```python
from build123d import *

# Parameters (mm, degrees)
F0_W     = 16
F0_H     = 8
F1_DEPTH = 8
F2_W     = 16
F2_H     = 3
F3_DEPTH = 33.2
F4_W     = 19
F4_H     = 3
F5_DEPTH = 12
F6_R     = 2
F7_DEPTH = 3
F8_W     = 16
F8_H     = 3
F9_DEPTH = 6
F10_R    = 1.99999


# Not quite as in the source:
# - a fillet or chamfer is up to 0.001 mm smaller than in the source, because OpenCascade refuses the exact size


with BuildPart() as f1:
    # F0 (on Top) → F1 (new body)
    with BuildSketch(Plane.XY):
        with Locations((-8, 4)):
            Rectangle(F0_W, F0_H)
    extrude(amount=F1_DEPTH)

    # F2 (on Top) → F3 (join)
    with BuildSketch(Plane.XY):
        with Locations((-8, -1.5)):
            Rectangle(F2_W, F2_H)
        Polygon((0, 6), (0, 0), (0, -3), (3, -3), (3, 6), align=None)
    extrude(amount=F3_DEPTH)

    # F4 (on face) → F5 (join)
    with BuildSketch(Plane.XZ.offset(3)):
        with Locations((-6.5, 1.5)):
            Rectangle(F4_W, F4_H)
    extrude(amount=F5_DEPTH)

    # F6 (on face) → F7 (cut, through all)
    with BuildSketch(Plane.XY.offset(3)):
        with Locations((-6.3249543309, -9.8292976618)):
            Circle(F6_R)
    extrude(amount=-F7_DEPTH, mode=Mode.SUBTRACT)

    # F8 (on face) → F9 (join)
    with BuildSketch(Plane(origin=(0, 0, 0), x_dir=(-1, 0, 0), z_dir=(0, 1, 0))):
        with Locations((8, 31.7)):
            Rectangle(F8_W, F8_H)
    extrude(amount=F9_DEPTH)

    # F10 (radius 2 in the source; OpenCascade refuses exactly that, so slightly less here)
    f10_edges = [f1.edges().sort_by_distance(p)[0] for p in [
        (-16, 6, 31.7),
        (-16, 8, 4),
        (0, 8, 4),
        (3, 6, 16.6),
        (3, -15, 1.5),
        (3, -3, 18.1),
        (-16, -3, 18.1),
        (-16, -15, 1.5),
    ]]
    fillet(f10_edges, radius=F10_R)


solid = f1.part
```
Verification items for the finished model (mm, model axes). A direction names the side the tool comes from. Round coordinates to 2 decimals unless told otherwise and drop trailing zeros. Order: outer loops, then holes, each group sorted by start corner. A loop starts at its lowest first (then second) coordinate and runs counter-clockwise, first axis right, second up. Notation, with made-up numbers: (76.25, 82) -> (82.25, 82) arc R17 cw to (82.25, 112) -> close; hole circle Ø10 at (-19, 42). An arc over 180 degrees is marked (long way). Put each result on its own line as item: value. Start each with the question number.
(1) Section check A-A (z = 13). Enter the section's corners in (x, y).
(2) Material ranges on line 1 along Z through (x, y) = (-3.5, 3.25); line 2 along Y through (x, z) = (0.5, 26); line 3 along Y through (x, z) = (-13.5, 22), recorded low to high.
(3) Section check B-B (x = -11). Enter the section's corners in (y, z).
(4) Section check C-C (y = 1.25). Enter the section's corners in (x, z), then the cut area to 3 significant figures.
(5) Draft check along Z on faces 4 (the face through (-0.57, 7.4, 4.06)), 5 (the face through (-8, 0, 19)), 6 (the face through (-9, -8, 3)). Enter one of: +Z half, -Z half, draft (parallel to the pull), parting line (faces both ways), or undercut.
(6) Tool access check on faces 1 (the face through (-15.4, -2.43, 18.31)), 2 (the face through (-7, -3, 18)), 3 (the face through (-15.4, 5.43, 31.72)). Record the directions out of +Z, -Z, +X, -X, +Y, -Y that give a thin tool (end or side, any length) a straight path to the whole face; none if there is none.
(7) Depth check by flat-ended pin: pin 1 Ø8 at (x, z) = (-10.5, 27) entering from -Y; pin 2 Ø4.5 at (x, z) = (-5, 23.5) entering from +Y; pin 3 Ø3 at (x, y) = (-8, 3.5) entering from -Z; pin 4 Ø3 at (y, z) = (4.5, 15.5) entering from -X. Enter the tip coordinate at first touch or a pass-through.
(8) Section check D-D (x = -6). Enter the section's corners in (y, z), then the cut area to 3 significant figures.
Completed:
1. outline: (-16, -1) arc R2 ccw to (-14, -3) -> (1, -3) arc R2 ccw to (3, -1) -> (3, 4) arc R2 ccw to (1, 6) -> (0, 6) -> (0, 0) -> (-16, 0) -> close
2. line 1: z = 0 to 8, 30.2 to 33.2
2. line 2: y = -3 to 6
2. line 3: y = -3 to 0
3. outline: (-15, 0) -> (8, 0) -> (8, 8) -> (0, 8) -> (0, 30.2) -> (6, 30.2) -> (6, 33.2) -> (-3, 33.2) -> (-3, 3) -> (-15, 3) -> close
4. outline: (-16, 0) -> (3, 0) -> (3, 33.2) -> (-16, 33.2) -> (-16, 30.2) -> (0, 30.2) -> (0, 8) -> (-16, 8) -> close
4. area: 276 mm2
5. face 4: draft
5. face 5: undercut
5. face 6: +Z half
6. face 1: +Z, -X, -Y
6. face 2: +Z, +X, -X, -Y
6. face 3: +Z, -X, +Y
7. pin 1: stops at y = -3
7. pin 2: stops at y = 0
7. pin 3: stops at z = 0
7. pin 4: stops at x = 0
8. outline: (-15, 0) -> (-11.8, 0) -> (-11.8, 3) -> (-15, 3) -> close; (-7.86, 0) -> (8, 0) -> (8, 8) -> (0, 8) -> (0, 30.2) -> (6, 30.2) -> (6, 33.2) -> (-3, 33.2) -> (-3, 3) -> (-7.86, 3) -> close
8. area: 206 mm2
